from build123d import *

# Parameters (mm, degrees)
EXTRUDE_1_DEPTH     = 4.5
EXTRUDE_2_DEPTH     = 7.4
SKETCH_3_R          = 11
EXTRUDE_3_DEPTH     = 4
CUT_EXTRUDE_2_REACH = 77.071
SKETCH_7_R          = 1.75


with BuildPart() as part:
    # 草图1 → 凸台-拉伸1 (new body)
    with BuildSketch(Plane.XY):
        with BuildLine():
            Line((-52.25, 0), (52.25, 0))
            ThreePointArc((52.25, 0), (0, -52.25), (-52.25, 0))
        make_face()
    extrude(amount=EXTRUDE_1_DEPTH)

    # 草图2 → 凸台-拉伸2 (add, symmetric)
    with BuildSketch(Plane.XY.offset(2.25)):
        with BuildLine():
            Line((-52.25, 0), (52.25, 0))
            ThreePointArc((52.25, 0), (52.22844668, -1.500619011), (52.163804501, -3))
            Line((52.163804501, -3), (-52.163804501, -3))
            ThreePointArc((-52.163804501, -3), (-52.22844668, -1.500619011), (-52.25, 0))
        make_face()
    extrude(amount=EXTRUDE_2_DEPTH, both=True)

    # 草图3 → 凸台-拉伸3 (add)
    with BuildSketch(Plane(origin=(0, -52.25, 0), x_dir=(1, 0, 0), z_dir=(0, 1, 0))):
        with Locations(Location((0, -2.25, 0), (0, 0, 168.19710831))):
            Circle(SKETCH_3_R)
    extrude(amount=EXTRUDE_3_DEPTH)

    # 草图7 → 切除-拉伸2 (cut, up to next)
    with BuildSketch(Plane.XZ.offset(52.25), mode=Mode.PRIVATE) as cut_extrude_2_sk1:
        with Locations(Location((0, 9.25, 0), (0, 0, 270))):
            Circle(SKETCH_7_R)
    cut_extrude_2_tool1 = extrude(cut_extrude_2_sk1.sketch, amount=-CUT_EXTRUDE_2_REACH, mode=Mode.PRIVATE) & part.part
    # 草图7 → 切除-拉伸2 (cut, up to next)
    with BuildSketch(Plane.XZ.offset(52.25), mode=Mode.PRIVATE) as cut_extrude_2_sk2:
        with Locations(Location((0, -4.75, 0), (0, 0, 270))):
            Circle(SKETCH_7_R)
    cut_extrude_2_tool2 = extrude(cut_extrude_2_sk2.sketch, amount=-CUT_EXTRUDE_2_REACH, mode=Mode.PRIVATE) & part.part
    add(cut_extrude_2_tool1.solids().sort_by_distance((0, -52.25, 9.25))[0], mode=Mode.SUBTRACT)
    add(cut_extrude_2_tool2.solids().sort_by_distance((0, -52.25, -4.75))[0], mode=Mode.SUBTRACT)


solid = part.part
Check sheet for the modelled part. Datum: model origin and axes. Units: mm. A direction names the side the tool comes from. Round coordinates to 2 decimals unless told otherwise and drop trailing zeros. Loops run counter-clockwise (first coordinate to the right, second up) from the corner with the lowest first, then second, coordinate; pieces in that order, holes last. Notation, with made-up numbers: M 36.5,22.25 L 83.5,22.25 A9 ccw 83.5,27.25 Z; hole C 58.5,-6 d5. An arc over 180 degrees is marked long. One line per question, with ' | ' between items. Start each with the question number.
Item 1: Release check for a two-part mould opening along Y. For faces 5 (the face through (1, -21, 0)), 6 (the face through (0, -52.25, 2)), 7 (the face through (0, -50, -3)) record: released by +Y, released by -Y, zero draft, split by the parting line, or undercut.
Item 2: Section check D-D (y = -27). Record the boundary of the cut face in (x, z).
Item 3: Section check C-C (z = 2.25). Record the boundary of the cut face in (x, y).
Item 4: Section check A-A (x = 0). Record the boundary of the cut face in (y, z), and give its area (3 significant figures).
Item 5: Gauge pin test, flat ends, axial feed: pin 1 Ø3.5 at (x, y) = (20, -2) entering from +Z; pin 2 Ø8 at (y, z) = (-38, 4) entering from -X; pin 3 Ø2 at (x, y) = (-21.5, -17.5) entering from +Z. Record the tip position at first contact, or that the pin passes through.
Item 6: Scan lines: probe 1 along Y at (x, z) = (7, -1); probe 2 along Y at (x, z) = (3.5, 11); probe 3 along X at (y, z) = (-50.6, 9.25). Record each from-to range of solid material in increasing order.
Item 7: Section check B-B (x = 13). Record the boundary of the cut face in (y, z), and give its area (3 significant figures).
Item 8: Set-up check for faces 1 (the face through (1, -48.25, -3)), 2 (the face through (0, -48.25, 7)), 3 (the face through (-0.67, -50.278, 7.633)), 4 (the face through (-1, 0, 2)): record each of +Z, -Z, +X, -X, +Y, -Y from which the full face is reachable in a straight line by a thin tool's end or side.
Worked out:
1) face 5: undercut | face 6: released by -Y | face 7: zero draft
2) outline: M -44.73,0 L 44.73,0 L 44.73,4.5 L -44.73,4.5 Z
3) outline: M -52.25,0 A52.25 ccw -11,-51.08 L -11,-52.25 L 11,-52.25 L 11,-51.08 A52.25 ccw 52.25,0 Z
4) outline: M -52.25,-8.75 L -48.25,-8.75 L -48.25,-6.5 L -52.25,-6.5 Z; M -52.25,-3 L -48.25,-3 L -48.25,0 L -3,0 L -3,-5.15 L 0,-5.15 L 0,9.65 L -3,9.65 L -3,4.5 L -48.25,4.5 L -48.25,7.5 L -52.25,7.5 Z; M -52.25,11 L -48.25,11 L -48.25,13.25 L -52.25,13.25 Z | area: 308 mm^2
5) pin 1: z = 9.65 | pin 2: x = -39.67 | pin 3: z = 4.5
6) probe 1: -52.25 to -48.25, -3 to 0 | probe 2: -52.25 to -48.25 | probe 3: -8.49 to -1.75, 1.75 to 8.49
7) outline: M -50.61,0 L -3,0 L -3,-5.15 L 0,-5.15 L 0,9.65 L -3,9.65 L -3,4.5 L -50.61,4.5 Z | area: 259 mm^2
8) face 1: -Z, +X, -X | face 2: +Z, +X, -X | face 3: -Y | face 4: +Z, -Z, +X, -X, +Y
